```python
from build123d import *

# Parameters (mm, degrees)
F0_W     = 203.2
F0_H     = 254
F0_R     = 2.38125
F0_R_2   = 19.05
F0_W_2   = 12.7
F0_H_2   = 6.35
F0_W_3   = 6.35
F0_H_3   = 12.7
F0_H_4   = 6.567365
F0_W_4   = 50.8
F0_H_5   = 50.8
F1_DEPTH = 6.35


with BuildPart() as f1:
    # F0 (on Top) → F1 (new body)
    with BuildSketch(Plane.XY):
        with Locations((101.6, 127)):
            Rectangle(F0_W, F0_H)
        with Locations((73.025, 60.325)):
            Circle(F0_R, mode=Mode.SUBTRACT)
        with Locations((101.6, 88.9)):
            Circle(F0_R_2, mode=Mode.SUBTRACT)
        with Locations((73.025, 117.475)):
            Circle(F0_R, mode=Mode.SUBTRACT)
        with Locations((130.175, 60.325)):
            Circle(F0_R, mode=Mode.SUBTRACT)
        with Locations((130.175, 117.475)):
            Circle(F0_R, mode=Mode.SUBTRACT)
        with Locations((12.7, 187.325)):
            Rectangle(F0_W_2, F0_H_2, mode=Mode.SUBTRACT)
        with Locations((44.45, 187.325)):
            Rectangle(F0_W_2, F0_H_2, mode=Mode.SUBTRACT)
        with Locations((60.325, 187.325)):
            Rectangle(F0_W_3, F0_H_2, mode=Mode.SUBTRACT)
        with Locations((12.7, 244.475)):
            Rectangle(F0_W_2, F0_H_2, mode=Mode.SUBTRACT)
        with Locations((44.45, 244.475)):
            Rectangle(F0_W_2, F0_H_2, mode=Mode.SUBTRACT)
        with Locations((53.975, 203.2)):
            Rectangle(F0_W_3, F0_H_3, mode=Mode.SUBTRACT)
        with Locations((60.325, 215.791317)):
            Rectangle(F0_W_3, F0_H_4, mode=Mode.SUBTRACT)
        with Locations((101.6, 215.9)):
            Rectangle(F0_W_4, F0_H_5, mode=Mode.SUBTRACT)
        with Locations((53.975, 228.6)):
            Rectangle(F0_W_3, F0_H_3, mode=Mode.SUBTRACT)
        with Locations((60.325, 244.475)):
            Rectangle(F0_W_3, F0_H_2, mode=Mode.SUBTRACT)
        with Locations((142.875, 187.325)):
            Rectangle(F0_W_3, F0_H_2, mode=Mode.SUBTRACT)
        with Locations((158.75, 187.325)):
            Rectangle(F0_W_2, F0_H_2, mode=Mode.SUBTRACT)
        with Locations((190.5, 187.325)):
            Rectangle(F0_W_2, F0_H_2, mode=Mode.SUBTRACT)
        with Locations((149.225, 203.2)):
            Rectangle(F0_W_3, F0_H_3, mode=Mode.SUBTRACT)
        with Locations((142.875, 215.791317)):
            Rectangle(F0_W_3, F0_H_4, mode=Mode.SUBTRACT)
        with Locations((149.225, 228.6)):
            Rectangle(F0_W_3, F0_H_3, mode=Mode.SUBTRACT)
        with Locations((142.875, 244.475)):
            Rectangle(F0_W_3, F0_H_2, mode=Mode.SUBTRACT)
        with Locations((158.75, 244.475)):
            Rectangle(F0_W_2, F0_H_2, mode=Mode.SUBTRACT)
        with Locations((190.5, 244.475)):
            Rectangle(F0_W_2, F0_H_2, mode=Mode.SUBTRACT)
    extrude(amount=F1_DEPTH)


solid = f1.part
```
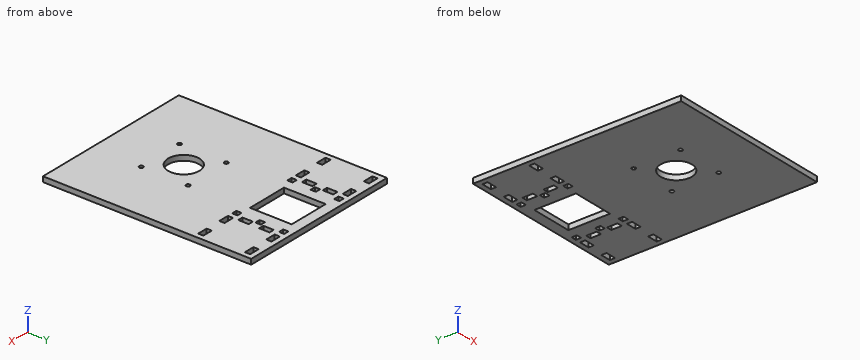
Here's how the part is built. I have some questions about the finished solid (model axes, mm). Coordinates: 2 decimals unless noted, no trailing zeros. Write each loop counter-clockwise with the first axis right and the second up, starting at its lowest first coordinate (ties: lowest second). Pieces come first, ordered by that corner, then holes. Notation, with made-up numbers: (53, 13.25) - (110, 13.25) arc R18 cw to (110, 39.25) - close; hole circle Ø6 at (59.5, 53.5). An arc over 180 degrees is marked (long way). One line per item, written item: value.
1) Suppose I cut it at B-B on y = 88.9. Write out the boundary of the cut face in (x, z).
Model answer:
outline: (0, 0) - (82.55, 0) - (82.55, 6.35) - (0, 6.35) - close; (120.65, 0) - (203.2, 0) - (203.2, 6.35) - (120.65, 6.35) - close
2) Suppose I cut it at A-A on x = 156.5. Write out the boundary of the cut face in (y, z), and give its area (3 significant figures).
Model answer:
outline: (0, 0) - (184.15, 0) - (184.15, 6.35) - (0, 6.35) - close; (190.5, 0) - (241.3, 0) - (241.3, 6.35) - (190.5, 6.35) - close; (247.65, 0) - (254, 0) - (254, 6.35) - (247.65, 6.35) - close
area: 1,530 mm²
3) I need wall thicknesses on line 1 along Y through (x, z) = (147, 4); line 2 along Y through (x, z) = (140, 1.75) (3 decimals); line 3 along Y through (x, z) = (153.5, 6). Which ranges of each line are inside material? Lowest first, please.
Model answer:
line 1: y = 0 to 196.85, 209.55 to 222.25, 234.95 to 254
line 2: y = 0 to 184.15, 190.5 to 212.508, 219.075 to 241.3, 247.65 to 254
line 3: y = 0 to 184.15, 190.5 to 241.3, 247.65 to 254
4) Suppose I cut it at D-D on z = 3.5. State how many separate pieces and enclosed holes the cut face has, and give its area (3 significant figures).
Model answer:
separate pieces: 1
enclosed holes: 24
area: 46,600 mm²
5) Suppose I cut it at C-C on x = 101.6. Write out the boundary of the cut face in (y, z), and give its area (3 significant figures).
Model answer:
outline: (0, 0) - (69.85, 0) - (69.85, 6.35) - (0, 6.35) - close; (107.95, 0) - (190.5, 0) - (190.5, 6.35) - (107.95, 6.35) - close; (241.3, 0) - (254, 0) - (254, 6.35) - (241.3, 6.35) - close
area: 1,050 mm²
